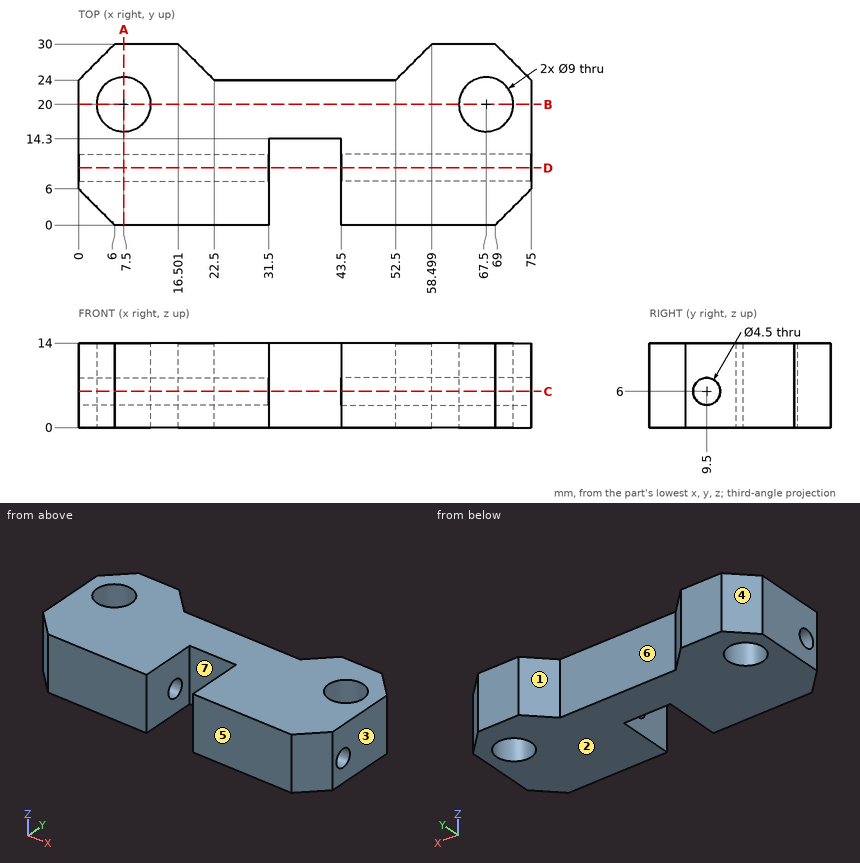
The figure shows three views and two pictorial views of one solid part (mm, origin at its lowest corner). Answer the questions. A direction names the side the tool comes from. Give positions to 0.01 mm unless a question says otherwise; leave off trailing zeros. Loops run counter-clockwise (first coordinate to the right, second up) from the corner with the lowest first, then second, coordinate; pieces in that order, holes last. Notation, with made-up numbers: (68.25, 66) - (107.25, 66) arc R16 ccw to (107.25, 95) - close; hole circle Ø3 at (-15, 29). An arc over 180 degrees is marked (long way). Answer in a Markdown table with one row per item.
(1) Flat-ended cylindrical pins translate along their axes: pin 1 Ø4 at (x, z) = (42.5, 6) entering from +Y; pin 2 Ø7 at (y, z) = (4, 7.5) entering from -X; pin 3 Ø1.5 at (x, y) = (10.5, 21) entering from +Z; pin 4 Ø1 at (x, z) = (38.5, 7) entering from -Y. Find the tip coordinate at first contact, or state that the pin passes through.
Results list:
| item | result |
|---|---|
| pin 1 | stops at y = 24 |
| pin 2 | stops at x = 0 |
| pin 3 | passes through |
| pin 4 | stops at y = 14.3 |
(2) For a pull along X with two mould halves and no side action, classify the marked faces 1, 2, 3 and 4 as pulls with the +X half, pulls with the -X half, needs draft (parallel to the pull), parting line crosses it, or undercut.
Results list:
| item | result |
|---|---|
| face 1 | undercut |
| face 2 | needs draft |
| face 3 | pulls with the +X half |
| face 4 | pulls with the -X half |
(3) Consider L1, parallel to X at y = 14, z = 8.75; L2, parallel to Y at x = 67.5, z = 9.25; L3, parallel to Y at x = 7.5, z = 6.5 (1 decimal). Determine where each line is inside the solid, lowest interval first. Write a range as [from, to].
Results list:
| item | result |
|---|---|
| L1 | x = [0, 31.5], [43.5, 75] |
| L2 | y = [0, 15.5], [24.5, 30] |
| L3 | y = [0, 7.3], [11.7, 15.5], [24.5, 30] |
(4) Section A-A (x = 7.5) is taken. Give the vertices of the cut face in (y, z).
Results list:
| item | result |
|---|---|
| outline | (0, 0) - (15.5, 0) - (15.5, 14) - (0, 14) - close; (24.5, 0) - (30, 0) - (30, 14) - (24.5, 14) - close; hole circle Ø4.5 at (9.5, 6) |
(5) Section D-D (y = 9.5) is taken. Give the vertices of the cut face in (x, z).
Results list:
| item | result |
|---|---|
| outline | (0, 0) - (31.5, 0) - (31.5, 3.75) - (0, 3.75) - close; (0, 8.25) - (31.5, 8.25) - (31.5, 14) - (0, 14) - close; (43.5, 0) - (75, 0) - (75, 3.75) - (43.5, 3.75) - close; (43.5, 8.25) - (75, 8.25) - (75, 14) - (43.5, 14) - close |
(6) A tool of negligible diameter and unlimited length cuts with its end or side. For the marked faces 5, 6 and 7, from which of +Z, -Z, +X, -X, +Y, -Y can it reach the whole face along a straight path? Write none if from no direction.
Results list:
| item | result |
|---|---|
| face 5 | +Z, -Z, +X, -X, -Y |
| face 6 | +Z, -Z, +Y |
| face 7 | +Z, -Z, -Y |
(7) Section B-B (y = 20) is taken. Give the vertices of the cut face in (x, z).
Results list:
| item | result |
|---|---|
| outline | (0, 0) - (3, 0) - (3, 14) - (0, 14) - close; (12, 0) - (63, 0) - (63, 14) - (12, 14) - close; (72, 0) - (75, 0) - (75, 14) - (72, 14) - close |
(8) Section C-C (z = 6) is taken. State how many separate pieces and enclosed holes the cut face has, and give its area (3 significant figures).
Results list:
| item | result |
|---|---|
| separate pieces | 3 |
| enclosed holes | 2 |
| area | 1,380 mm² |
